Read the model definition and answer for the solid it produces. Units are mm, in the model's axes. A direction names the side the tool comes from. Give positions to 0.01 mm unless a question says otherwise; leave off trailing zeros.
Item 1: Find the intervals of material crossed by line 1 along X through (y, z) = (11.5, -253); line 2 along Y through (x, z) = (5, -388.5), in increasing order.
Item 2: Which of the six approach directions +Z, -Z, +X, -X, +Y, -Y give full straight-line access (tool end or side, diameter ignored) to faces 4 (the face through (-10, 20, -246)), 5 (the face through (15, -11.25, -246))?
Item 3: A cutting plane is placed at A-A (z = -384). State how many separate pieces and enclosed holes the cut face has, plus the area to 3 significant figures.
Item 4: Given pin 1 Ø0.5 at (x, z) = (19.5, -177) entering from -Y; pin 2 Ø3 at (x, z) = (-0.5, -218.5) entering from -Y; pin 3 Ø0.8 at (x, z) = (-19.5, -201.5) entering from +Y, each flat-ended and moving along its own axis, determine where each tip first touches the part or whether it passes through.
Item 5: The mould has two halves that part along X. Classify faces 1 (the face through (11.25, 15, -246)), 2 (the face through (10, 20, -246)), 3 (the face through (20, -10, -246)): +X half, -X half, draft (parallel to the pull), parting line (faces both ways), or undercut.
from build123d import *

# Parameters (mm, degrees)
SKETCH_1_W          = 40
SKETCH_1_H          = 40
EXTRUDE_1_DEPTH     = 500
CUT_EXTRUDE_1_DEPTH = 501
SKETCH_3_W          = 7.75
SKETCH_3_H          = 7.75
CUT_EXTRUDE_2_DEPTH = 501
SKETCH_4_R          = 3.4
CUT_EXTRUDE_3_DEPTH = 501
FILLET_1_R          = 4.5


with BuildPart() as part:
    # 草图1 → 凸台-拉伸1 (new body)
    with BuildSketch(Plane.XY):
        Rectangle(SKETCH_1_W, SKETCH_1_H)
    extrude(amount=-EXTRUDE_1_DEPTH)

    # 草图2 → 切除-拉伸1 (cut, through all)
    with BuildSketch(Plane.XY):
        Polygon((-19, 5.1), (-20, 5.1), (-20, -5.1), (-19, -5.1), (-19, -4.1), (-15.6, -4.1), (-15.6, -6.1), (-18, -6.1), (-18, -10.25), (-11.38137085, -10.25), (-5.5, -4.36862915), (-5.5, 4.36862915), (-11.38137085, 10.25), (-18, 10.25), (-18, 6.1), (-15.6, 6.1), (-15.6, 4.1), (-19, 4.1), align=None)
        Polygon((-5.1, -19), (-5.1, -20), (5.1, -20), (5.1, -19), (4.1, -19), (4.1, -15.6), (6.1, -15.6), (6.1, -18), (10.25, -18), (10.25, -11.38137085), (4.36862915, -5.5), (-4.36862915, -5.5), (-10.25, -11.38137085), (-10.25, -18), (-6.1, -18), (-6.1, -15.6), (-4.1, -15.6), (-4.1, -19), align=None)
        Polygon((20, -5.1), (20, 5.1), (19, 5.1), (19, 4.1), (15.6, 4.1), (15.6, 6.1), (18, 6.1), (18, 10.25), (11.38137085, 10.25), (5.5, 4.36862915), (5.5, -4.36862915), (11.38137085, -10.25), (18, -10.25), (18, -6.1), (15.6, -6.1), (15.6, -4.1), (19, -4.1), (19, -5.1), align=None)
        Polygon((5.1, 20), (-5.1, 20), (-5.1, 19), (-4.1, 19), (-4.1, 15.6), (-6.1, 15.6), (-6.1, 18), (-10.25, 18), (-10.25, 11.38137085), (-4.36862915, 5.5), (4.36862915, 5.5), (10.25, 11.38137085), (10.25, 18), (6.1, 18), (6.1, 15.6), (4.1, 15.6), (4.1, 19), (5.1, 19), align=None)
    extrude(amount=-CUT_EXTRUDE_1_DEPTH, mode=Mode.SUBTRACT)

    # 草图3 → 切除-拉伸2 (cut, through all)
    with BuildSketch(Plane.XY):
        with Locations((-15.125, 15.125)):
            Rectangle(SKETCH_3_W, SKETCH_3_H)
        with Locations((15.125, 15.125)):
            Rectangle(SKETCH_3_W, SKETCH_3_H)
        with Locations((15.125, -15.125)):
            Rectangle(SKETCH_3_W, SKETCH_3_H)
        with Locations((-15.125, -15.125)):
            Rectangle(SKETCH_3_W, SKETCH_3_H)
    extrude(amount=-CUT_EXTRUDE_2_DEPTH, mode=Mode.SUBTRACT)

    # 草图4 → 切除-拉伸3 (cut, through all)
    with BuildSketch(Plane.XY):
        Circle(SKETCH_4_R)
    extrude(amount=-CUT_EXTRUDE_3_DEPTH, mode=Mode.SUBTRACT)

    # 圆角1
    fillet_1_edges = [part.edges().sort_by_distance(p)[0] for p in [
        (-19, -19, -250),
        (19, -19, -250),
        (19, 19, -250),
        (-19, 19, -250),
        (20, -20, -250),
        (-20, -20, -250),
        (-20, 20, -250),
        (20, 20, -250),
    ]]
    fillet(fillet_1_edges, radius=FILLET_1_R)


solid = part.part
Response values:
1. line 1: x = -20 to -19, -11.25 to -10.25, 10.25 to 11.25, 19 to 20
1. line 2: y = -19 to -15.6, -6.13 to 6.13, 15.6 to 19
2. face 4: +Z, -Z, +X, -X, +Y
2. face 5: +Z, -Z
3. separate pieces: 1
3. enclosed holes: 5
3. area: 402 mm2
4. pin 1: stops at y = -17.99
4. pin 2: stops at y = -5.5
4. pin 3: stops at y = 18.2
5. face 1: undercut
5. face 2: draft
5. face 3: +X half
